Design review of the part built by this model. Coordinates are the model's own, in mm. A direction names the side the tool comes from. Coordinates: 2 decimals unless noted, no trailing zeros. Write each loop counter-clockwise with the first axis right and the second up, starting at its lowest first coordinate (ties: lowest second). Pieces come first, ordered by that corner, then holes. Notation, with made-up numbers: (24, 51) -> (65, 51) arc R22 ccw to (65, 88) -> close; hole circle Ø5 at (6.5, 54.5). An arc over 180 degrees is marked (long way). Return JSON: item names as keys, results as strings. Group by question number.
from build123d import *

# Parameters (mm, degrees)
SKETCH1_R           = 70
BOSS_EXTRUDE1_DEPTH = 17
SKETCH2_R           = 7.5
CUT_EXTRUDE1_DEPTH  = 101.444014257
SKETCH3_R           = 5.906037177
CUT_EXTRUDE2_DEPTH  = 14.09728
CIRPATTERN1_START   = 2.902719908
CIRPATTERN1_DEPTH   = 14.097280092


# Read off the part's stored shape, not the designer's step: CirPattern1
with BuildPart() as part:
    # Sketch1 → Boss-Extrude1 (new body)
    with BuildSketch(Plane(origin=(0, 0, 0), x_dir=(1, 0, 0), z_dir=(0, 1, 0))):
        with Locations(Location((0, 0, 0), (0, 0, 270))):
            Circle(SKETCH1_R)
    extrude(amount=BOSS_EXTRUDE1_DEPTH)

    # Sketch2 → Cut-Extrude1 (cut, through all)
    with BuildSketch(Plane(origin=(0, 0, 0), x_dir=(1, 0, 0), z_dir=(0, 1, 0))):
        with Locations(Location((0, 0, 0), (0, 0, 270))):
            Circle(SKETCH2_R)
    extrude(amount=CUT_EXTRUDE1_DEPTH, mode=Mode.SUBTRACT)

    # Sketch3 → Cut-Extrude2 (cut)
    with BuildSketch(Plane(origin=(0, 17, 0), x_dir=(1, 0, 0), z_dir=(0, 1, 0))):
        with Locations((-9.676366693, 0)):
            Circle(SKETCH3_R)
    extrude(amount=-CUT_EXTRUDE2_DEPTH, mode=Mode.SUBTRACT)

    # CirPattern1 outline → CirPattern1 (cut)
    with BuildSketch(Plane(origin=(0, 0, 0), x_dir=(1, 0, 0), z_dir=(0, 1, 0)).offset(CIRPATTERN1_START)):
        with BuildLine():
            ThreePointArc((-5.942354238, -4.575852501), (-9.13373708, -5.881056727), (-12.510062779, -5.181837669))
            ThreePointArc((-12.510062779, -5.181837669), (-11.018423444, -11.018423444), (-5.181837669, -12.510062779))
            ThreePointArc((-5.181837669, -12.510062779), (0, -15.58240387), (5.181837669, -12.510062779))
            ThreePointArc((5.181837669, -12.510062779), (11.018423444, -11.018423444), (12.510062779, -5.181837669))
            ThreePointArc((12.510062779, -5.181837669), (15.58240387, 0), (12.510062779, 5.181837669))
            ThreePointArc((12.510062779, 5.181837669), (11.018423444, 11.018423444), (5.181837669, 12.510062779))
            ThreePointArc((5.181837669, 12.510062779), (0, 15.58240387), (-5.181837669, 12.510062779))
            ThreePointArc((-5.181837669, 12.510062779), (-11.018423444, 11.018423444), (-12.510062779, 5.181837669))
            ThreePointArc((-12.510062779, 5.181837669), (-9.13373708, 5.881056727), (-5.942354238, 4.575852501))
            ThreePointArc((-5.942354238, 4.575852501), (7.5, 0), (-5.942354238, -4.575852501))
        make_face()
    extrude(amount=CIRPATTERN1_DEPTH, mode=Mode.SUBTRACT)


solid = part.part
Q1. We need section C-C on y = 9.25. Write out the cut boundary in (x, z), plus the area to 3 significant figures.
Q2. We need section D-D on z = -23. Write out the cut boundary in (x, y), plus the area to 3 significant figures.
Q3. We need section A-A on x = 0. Write out the cut boundary in (y, z).
Q4. The part is to be moulded in two halves that separate along X. For faces 1 (the cylindrical face through (-42.594, 8.381, -55.55)), 2 (the cylindrical face through (15.58, 9.85, 0.09)), 3 (the flat face through (1, 17, -17)), say which applies: +X half, -X half, draft (parallel to the pull), parting line (faces both ways), or undercut.
Q5. For faces 4 (the cylindrical face through (-15.58, 10.05, -0.09)), 5 (the flat face through (-15, 0, -1)), list the 3-axis set-ups (+Z, -Z, +X, -X, +Y, -Y) from which the entire face can be reached by the end or side of a thin tool; tool diameter is ignored.
Q6. For P1, Ø3, axis at x = 45.5, z = -34, coming from the -Y side; P2, Ø2, axis at x = 32, y = 10.5, coming from the +Z side; P3, Ø10, axis at y = 4, z = 10.5, coming from the +X side; P4, Ø5, axis at x = -44.5, y = 6, coming from the -Z side, all flat-tipped, find the tip position at first contact; note any pin that passes through.
Q7. We need section B-B on z = 0. Write out the cut boundary in (x, y), plus the area to 3 significant figures.
Q8. Wall thickness on L1, parallel to X at y = 2.25, z = 0; L2, parallel to Z at x = 12, y = 9; L3, parallel to Z at x = -9.5, y = 15.75: over which ranges is each line inside the solid? List them lowest first.
Findings below:
{
 "1": {"outline": "circle Ø140 at (0, 0); hole (-12.51, -5.18) arc R5.91 ccw to (-5.18, -12.51) arc R5.91 ccw to (5.18, -12.51) arc R5.91 ccw to (12.51, -5.18) arc R5.91 ccw to (12.51, 5.18) arc R5.91 ccw to (5.18, 12.51) arc R5.91 ccw to (-5.18, 12.51) arc R5.91 ccw to (-12.51, 5.18) arc R5.91 ccw to start", "area": "14,700 mm^2"},
 "2": {"outline": "(-66.11, 0) -> (66.11, 0) -> (66.11, 17) -> (-66.11, 17) -> close", "area": "2,250 mm^2"},
 "3": {"outline": "(0, -70) -> (17, -70) -> (17, -15.58) -> (2.9, -15.58) -> (2.9, -7.5) -> (0, -7.5) -> close; (0, 7.5) -> (2.9, 7.5) -> (2.9, 15.58) -> (17, 15.58) -> (17, 70) -> (0, 70) -> close"},
 "4": {"face 1": "parting line", "face 2": "undercut", "face 3": "draft"},
 "5": {"face 4": "+Y", "face 5": "+Z, -Z, +X, -X, -Y"},
 "6": {"P1": "stops at y = 0", "P2": "stops at z = 62.76", "P3": "stops at x = 69.78", "P4": "stops at z = -56"},
 "7": {"outline": "(-70, 0) -> (-7.5, 0) -> (-7.5, 2.9) -> (-15.58, 2.9) -> (-15.58, 17) -> (-70, 17) -> close; (7.5, 0) -> (70, 0) -> (70, 17) -> (15.58, 17) -> (15.58, 2.9) -> (7.5, 2.9) -> close", "area": "1,900 mm^2"},
 "8": {"L1": "x = -70 to -7.5, 7.5 to 70", "L2": "z = -68.96 to -9.72, 9.72 to 68.96", "L3": "z = -69.35 to -12.12, 12.12 to 69.35"}
}
